Autodesk Inventor part; units mm, degrees
ref_plane "YZ Plane" through (0, 0, 0) normal (1, 0, 0) x (0, 1, 0)
ref_plane "XZ Plane" through (0, 0, 0) normal (0, 1, 0) x (-1, 0, 0)
ref_plane "XY Plane" through (0, 0, 0) normal (0, 0, 1) x (1, 0, 0)
sketch "Sketch1" plane through (0, 0, 0) normal (0, 0, 1) x (1, 0, 0)
  line L0 (-22, 20) -> (22, 20)
  line L1 (22, 20) -> (22, 0)
  line L2 (22, 0) -> (-22, 0)
  line L3 (-22, 0) -> (-22, 20)
  line L4 (-22, 20) -> (22, 0) construction
  line L5 (22, 20) -> (-22, 0) construction
  line L6 (-29, 2) -> (-22, 2)
  line L7 (-22, 2) -> (-22, 0)
  line L8 (-22, 0) -> (-29, 0)
  line L9 (-29, 0) -> (-29, 2)
  line L10 (-29, 2) -> (-22, 0) construction
  line L11 (-22, 2) -> (-29, 0) construction
  line L12 (29, 2) -> (22, 2)
  line L13 (22, 2) -> (22, 0)
  line L14 (22, 0) -> (29, 0)
  line L15 (29, 0) -> (29, 2)
  line L16 (29, 2) -> (22, 0) construction
  line L17 (22, 2) -> (29, 0) construction
  point P0 (0, 0)
  point P1 (0, 10)
  point P2 (-25.5, 1)
  point P3 (25.5, 1)
  dimension "d0" = 58
  dimension "d1" = 20
  dimension "d2" = 2
  dimension "d3" = 44
extrude "Extrusion1" add sketch "Sketch1" along normal mid plane 24
sketch "Sketch2" plane through (-29, 0, 12) normal (0, -1, 0) x (1, 0, 0)
  line L0 (58, -24) -> (58, 0)
  line L1 (51, -10) -> (58, -10)
  line L2 (58, -10) -> (58, -14)
  line L3 (58, -14) -> (51, -14)
  line L4 (51, -14) -> (51, -10)
  line L5 (51, -10) -> (58, -14) construction
  line L6 (58, -10) -> (51, -14) construction
  line L7 (0, -24) -> (0, 0)
  line L8 (7, -10) -> (0, -10)
  line L9 (0, -10) -> (0, -14)
  line L10 (0, -14) -> (7, -14)
  line L11 (7, -14) -> (7, -10)
  line L12 (7, -10) -> (0, -14) construction
  line L13 (0, -10) -> (7, -14) construction
  point P0 (29, -12)
  point P1 (54.5, -12)
  point P2 (3.5, -12)
  point P3 (0, -10)
  dimension "d6" = 4
  dimension "d7" = 44
extrude "Extrusion2" cut sketch "Sketch2" against normal blind 24
properties part number "DCDC24Vto15V"
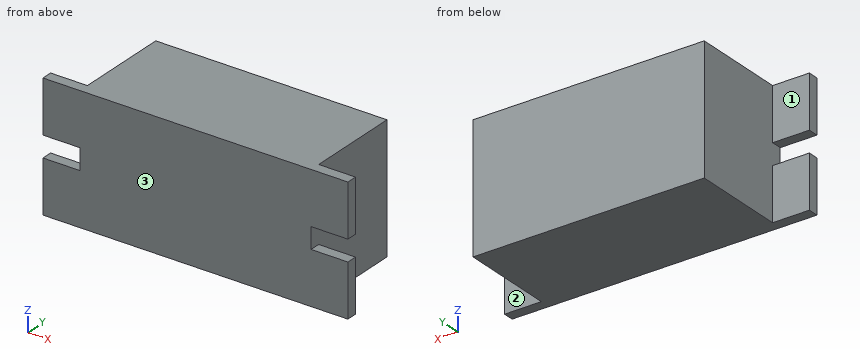
Verification items for the finished model (mm, model axes). Face numbers are marked on the shaded views. A direction names the side the tool comes from. Coordinates: 2 decimals unless noted, no trailing zeros. Loops run counter-clockwise (first coordinate to the right, second up) from the corner with the lowest first, then second, coordinate; pieces in that order, holes last. Notation, with made-up numbers: (-5.75, 22) -> (-0.75, 22) arc R24 cw to (-0.75, 32) -> close; hole circle Ø2 at (0.25, 69). An arc over 180 degrees is marked (long way). Answer in a Markdown table with one row per item. Add a question column.
1. Section check C-C, the plane y = 15.5. Enter the section's corners in (x, z).
2. Depth check by flat-ended pin: P1, Ø5.5, axis at x = -25, z = 7.5, coming from the +Y side; P2, Ø4, axis at y = 8.5, z = 0.5, coming from the -X side. Enter the tip coordinate at first touch or a pass-through.
3. Section check A-A, the plane x = 25.5. Enter the section's corners in (y, z).
4. Access from +Z, -Z, +X, -X, +Y, -Y to the whole of each face (thin tool, end or side, straight path). Record for the marked faces 1, 2 and 3.
5. Material ranges on probe 1 along X at (y, z) = (13.25, -6), recorded low to high. Write a range as [from, to].
6. Section check B-B, the plane z = -2.75. Enter the section's corners in (x, y), then the cut area to 3 significant figures.
Derived:
| question | item | result |
|---|---|---|
| 1 | outline | (-22, -12) -> (22, -12) -> (22, 12) -> (-22, 12) -> close |
| 2 | P1 | stops at y = 2 |
| 2 | P2 | stops at x = -22 |
| 3 | outline | (0, -12) -> (2, -12) -> (2, -2) -> (0, -2) -> close; (0, 2) -> (2, 2) -> (2, 12) -> (0, 12) -> close |
| 4 | face 1 | +Z, -Z, -X, +Y |
| 4 | face 2 | +Z, -Z, +X, +Y |
| 4 | face 3 | +Z, -Z, +X, -X, -Y |
| 5 | probe 1 | x = [-22, 22] |
| 6 | outline | (-29, 0) -> (29, 0) -> (29, 2) -> (22, 2) -> (22, 20) -> (-22, 20) -> (-22, 2) -> (-29, 2) -> close |
| 6 | area | 908 mm² |
